```python
from build123d import *

# Parameters (mm, degrees)
TROU_TARAUD_M31_D       = 2.5
TROU_TARAUD_M31_DEPTH   = 8.5
TROU_TARAUD_M31_TIP     = 0.751075774
ESQUISSE4_R             = 3
ESQUISSE4_R_2           = 2.5
ENL_V_MAT_EXTRU_1_DEPTH = 0.5


with BuildPart() as part:
    # Esquisse1 → Révolution1 (revolve)
    with BuildSketch(Plane.XY):
        Polygon((0, 0), (0, 2.5), (1, 2.5), (1, 2), (3, 2), (3, 3), (14, 3), (14, 0), align=None)
    revolve(axis=Axis((14, 0, 0), (-1, 0, 0)))

    # Trou taraudé M31
    with Locations(Plane(origin=(14, 0, 0), x_dir=(0, 0, -1), z_dir=(1, 0, 0))):
        with Locations((0, 0)):
            Hole(TROU_TARAUD_M31_D / 2, depth=TROU_TARAUD_M31_DEPTH)
            with Locations((0, 0, -(TROU_TARAUD_M31_DEPTH + TROU_TARAUD_M31_TIP / 2))):  # 118° drill point
                Cone(0, TROU_TARAUD_M31_D / 2, TROU_TARAUD_M31_TIP, mode=Mode.SUBTRACT)

    # Esquisse4 → Enlèv. mat.-Extru.1 (cut, symmetric)
    with BuildSketch(Plane.ZY.offset(-7.5)):
        Circle(ESQUISSE4_R)
        Circle(ESQUISSE4_R_2, mode=Mode.SUBTRACT)
    extrude(amount=ENL_V_MAT_EXTRU_1_DEPTH, both=True, mode=Mode.SUBTRACT)


solid = part.part
```
Can you work these out from the model? Positions are in its coordinate system, mm. A direction names the side the tool comes from. Coordinates: 2 decimals unless noted, no trailing zeros. Order: outer loops, then holes, each group sorted by start corner. A loop starts at its lowest first (then second) coordinate and runs counter-clockwise, first axis right, second up. Notation, with made-up numbers: (-31, 8.5) -> (22, 8.5) arc R13 ccw to (22, 33.5) -> close; hole circle Ø11 at (-14, 74.5). An arc over 180 degrees is marked (long way). Write each question's results on one line, items separated by ' | '.
Item 1: I want a section at C-C, the plane x = 2.75. Write out the boundary of the cut face in (y, z), then the cut area to 3 significant figures.
Results are:
outline: circle Ø4 at (0, 0) | area: 12.6 mm²
Item 2: I want a section at B-B, the plane z = -1.75. Write out the boundary of the cut face in (x, y).
Results are:
outline: (0, -1.79) -> (1, -1.79) -> (1, -0.97) -> (3, -0.97) -> (3, -2.44) -> (7, -2.44) -> (7, -1.79) -> (8, -1.79) -> (8, -2.44) -> (14, -2.44) -> (14, 2.44) -> (8, 2.44) -> (8, 1.79) -> (7, 1.79) -> (7, 2.44) -> (3, 2.44) -> (3, 0.97) -> (1, 0.97) -> (1, 1.79) -> (0, 1.79) -> close
Item 3: If we mould it in two halves opening along Y, with no side actions, what happens to faces 1 (the face through (9.69, -1.22, -0.27)), 2 (the face through (4.88, -0.21, 0.05)), 3 (the face through (3, -1, 2)), 4 (the face through (2, 0, 2))? For each: +Y half, -Y half, draft (parallel to the pull), parting line (faces both ways), or undercut.
Results are:
face 1: undercut | face 2: undercut | face 3: draft | face 4: parting line
Item 4: Which directions (+Z, -Z, +X, -X, +Y, -Y) give clear straight access to the entire face, cutting with the end or side of a thin tool? Please do faces 5 (the face through (14, 1, 1)), 6 (the face through (0.51, -0.54, 2.44)), 7 (the face through (8, 2, -2)).
Results are:
face 5: +Z, -Z, +X, +Y, -Y | face 6: -X | face 7: none
Item 5: I want a section at A-A, the plane y = -1.7. Write out the boundary of the cut face in (x, z).
Results are:
outline: (0, -1.83) -> (1, -1.83) -> (1, -1.05) -> (3, -1.05) -> (3, -2.47) -> (7, -2.47) -> (7, -1.83) -> (8, -1.83) -> (8, -2.47) -> (14, -2.47) -> (14, 2.47) -> (8, 2.47) -> (8, 1.83) -> (7, 1.83) -> (7, 2.47) -> (3, 2.47) -> (3, 1.05) -> (1, 1.05) -> (1, 1.83) -> (0, 1.83) -> close
Item 6: If I drill on line 1 along Y through (x, z) = (7.5, 0); line 2 along X through (y, z) = (-1.6, 1.8); line 3 along Y through (x, z) = (9.5, 0), over which ranges is the centre line in solid material (lowest first)?
Results are:
line 1: -2.5 to -1.25, 1.25 to 2.5 | line 2: 0 to 1, 3 to 14 | line 3: -3 to -1.25, 1.25 to 3
Item 7: I'm going to push flat-ended pins straight in: pin 1 Ø1.5 at (y, z) = (0, 0) entering from +X; pin 2 Ø1.5 at (x, y) = (4.5, 1) entering from +Z; pin 3 Ø1.8 at (y, z) = (0.5, 1.5) entering from -X; pin 4 Ø2 at (x, z) = (9.5, -2.5) entering from +Y. Where does each tip first touch, or does it pass through?
Results are:
pin 1: x = 5.2 | pin 2: z = 2.99 | pin 3: x = 0 | pin 4: y = 2.6
Item 8: I want a section at D-D, the plane x = 8.5. Write out the boundary of the cut face in (y, z).
Results are:
outline: circle Ø6 at (0, 0); hole circle Ø2.5 at (0, 0)
